Source: CAD feature listing. Evaluate the final solid. Frame: model axes, mm. A direction names the side the tool comes from. Give positions to 0.01 mm unless a question says otherwise; leave off trailing zeros. Order: outer loops, then holes, each group sorted by start corner. A loop starts at its lowest first (then second) coordinate and runs counter-clockwise, first axis right, second up.
```python
from build123d import *

# Parameters (mm, degrees)
SKETCH1_W           = 34
SKETCH1_H           = 24
SKETCH1_W_2         = 30
SKETCH1_H_2         = 5
SKETCH1_W_3         = 5
SKETCH1_H_3         = 26
SKETCH1_W_4         = 40
BOSS_EXTRUDE1_DEPTH = 5
BOSS_EXTRUDE2_DEPTH = 13
SKETCH2_W           = 46
SKETCH2_H           = 32
BOSS_EXTRUDE6_DEPTH = 5


with BuildPart() as part:
    # Sketch1 → Boss-Extrude1 (new body)
    with BuildSketch(Plane.XY):
        Polygon((16, 52), (18, 52), (48, 52), (50, 52), (55, 52), (55, 57), (55, 59), (55, 79), (55, 81), (55, 86), (50, 86), (48, 86), (18, 86), (16, 86), (11, 86), (11, 81), (11, 79), (11, 59), (11, 57), (11, 52), align=None)
        with Locations((33, 69)):
            Rectangle(SKETCH1_W, SKETCH1_H, mode=Mode.SUBTRACT)
        Polygon((0, 91), (0, 52), (6, 52), (6, 59), (11, 59), (11, 79), (6, 79), (6, 91), align=None)
        with Locations((33, 88.5)):
            Rectangle(SKETCH1_W_2, SKETCH1_H_2)
        Polygon((60, 52), (66, 52), (66, 91), (60, 91), (60, 79), (55, 79), (55, 59), (60, 59), align=None)
        with Locations((63.5, 26)):
            Rectangle(SKETCH1_W_3, SKETCH1_H_3)
        with Locations((33, 49.5)):
            Rectangle(SKETCH1_W_2, SKETCH1_H_2)
        with Locations((2.5, 26)):
            Rectangle(SKETCH1_W_3, SKETCH1_H_3)
        with Locations((33, 2.5)):
            Rectangle(SKETCH1_W_4, SKETCH1_H_2)
    extrude(amount=BOSS_EXTRUDE1_DEPTH)

    # Sketch1_3 → Boss-Extrude2 (add)
    with BuildSketch(Plane.XY):
        Polygon((0, 42), (0, 39), (5, 39), (5, 47), (18, 47), (18, 52), (16, 52), (11, 52), (11, 57), (11, 59), (6, 59), (6, 52), (0, 52), (0, 47), align=None)
        Polygon((11, 91), (6, 91), (6, 79), (11, 79), (11, 81), (11, 86), (16, 86), (18, 86), (18, 91), align=None)
        Polygon((55, 91), (48, 91), (48, 86), (50, 86), (55, 86), (55, 81), (55, 79), (60, 79), (60, 91), align=None)
        Polygon((61, 47), (61, 39), (66, 39), (66, 42), (66, 47), (66, 52), (60, 52), (60, 59), (55, 59), (55, 57), (55, 52), (50, 52), (48, 52), (48, 47), align=None)
        Polygon((53, 5), (53, 0), (61, 0), (66, 0), (66, 5), (66, 13), (61, 13), (61, 5), align=None)
        Polygon((0, 5), (0, 0), (5, 0), (13, 0), (13, 5), (5, 5), (5, 13), (0, 13), align=None)
    extrude(amount=BOSS_EXTRUDE2_DEPTH)

    # Sketch2 → Boss-Extrude6 (add)
    with BuildSketch(Plane.XY.offset(5)):
        Polygon((5, 10), (5, 5), (10, 5), (13, 5), (53, 5), (56, 5), (61, 5), (61, 10), (61, 42), (61, 47), (56, 47), (10, 47), (5, 47), (5, 42), align=None)
        with Locations((33, 26)):
            Rectangle(SKETCH2_W, SKETCH2_H, mode=Mode.SUBTRACT)
    extrude(amount=-BOSS_EXTRUDE6_DEPTH)


solid = part.part
```
1) Reachability of faces 5 (the flat face through (8, 79, 9)), 6 (the flat face through (13, 2, 9)), 7 (the flat face through (48, 50, 9)), 8 (the flat face through (6, 85, 9)), 9 (the flat face through (56, 26, 3)) from +Z, -Z, +X, -X, +Y, -Y: full face, straight path, thin tool, end or side. Return the list, or none.
Report:
face 5: +Z, +X, -X
face 6: +Z, -Y
face 7: +Z, +Y, -Y
face 8: +Z, -X, +Y
face 9: +Z, -Z
2) Material intervals for L1, parallel to Y at x = 43, z = 1.25; L2, parallel to X at y = 40.5, z = 9.25; L3, parallel to Y at x = 50.5, z = 7.25, sorted ascending.
Report:
L1: y = 0 to 10, 42 to 57, 81 to 91
L2: x = 0 to 5, 61 to 66
L3: y = 47 to 52, 86 to 91
3) Section query A-A, the plane y = 23.5. Return the cut outline in (x, z), and give its area (3 significant figures).
Report:
outline: (0, 0) - (10, 0) - (10, 5) - (0, 5) - close; (56, 0) - (66, 0) - (66, 5) - (56, 5) - close
area: 100 mm2
4) Section query B-B, the plane x = 38.5. Return the cut outline in (y, z), and give its area (3 significant figures).
Report:
outline: (0, 0) - (10, 0) - (10, 5) - (0, 5) - close; (42, 0) - (57, 0) - (57, 5) - (42, 5) - close; (81, 0) - (91, 0) - (91, 5) - (81, 5) - close
area: 175 mm2
5) Draft query along X for faces 1 (the flat face through (6, 56, 9)), 2 (the flat face through (57, 5, 9)), 3 (the flat face through (33, 0, 4)), 4 (the flat face through (48, 89, 9)). Return one class per face: +X half, -X half, draft (parallel to the pull), parting line (faces both ways), or undercut.
Report:
face 1: -X half
face 2: undercut
face 3: draft
face 4: undercut
6) Section query D-D, the plane z = 2.25. Return the cut outline in (x, y).
Report:
outline: (0, 0) - (66, 0) - (66, 91) - (0, 91) - close; hole (10, 10) - (56, 10) - (56, 42) - (10, 42) - close; hole (16, 57) - (50, 57) - (50, 81) - (16, 81) - close
7) Pin query (flat end, axial travel): pin 1 (2.5 mm diameter, centred on y = 88.5, z = 9, fed in from -X); pin 2 (6 mm diameter, centred on x = 7.5, y = 26, fed in from +Z); pin 3 (5.5 mm diameter, centred on x = 63.5, z = 9, fed in from +Y). Return the tip coordinate at first contact, or that it passes through.
Report:
pin 1: stops at x = 6
pin 2: stops at z = 5
pin 3: stops at y = 52
8) Section query C-C, the plane x = 15. Return the cut outline in (y, z).
Report:
outline: (0, 0) - (10, 0) - (10, 5) - (0, 5) - close; (42, 0) - (91, 0) - (91, 13) - (86, 13) - (86, 5) - (52, 5) - (52, 13) - (47, 13) - (47, 5) - (42, 5) - close
